```python
from build123d import *

# Parameters (mm, degrees)
SKETCH15_R           = 11.5
BOSS_EXTRUDE8_DEPTH  = 8
BOSS_EXTRUDE9_START  = -8
SKETCH16_R           = 11.5
SKETCH16_R_2         = 11.3
BOSS_EXTRUDE9_DEPTH  = 8
SKETCH17_W           = 10
SKETCH17_H           = 3
BOSS_EXTRUDE10_DEPTH = 8
SKETCH18_W           = 8
SKETCH18_H           = 10
BOSS_EXTRUDE11_DEPTH = 2
SKETCH19_W           = 6
SKETCH19_H           = 3
CUT_EXTRUDE4_DEPTH   = 8
SKETCH20_R           = 2
CUT_EXTRUDE5_DEPTH   = 9
SKETCH21_W           = 29
SKETCH21_H           = 3
BOSS_EXTRUDE12_DEPTH = 7
SKETCH22_R           = 2
CUT_EXTRUDE6_DEPTH   = 7
FILLET1_R            = 5
SKETCH24_R           = 2
CUT_EXTRUDE10_DEPTH  = 8


with BuildPart() as part:
    # Sketch15 → Boss-Extrude8 (new body)
    with BuildSketch(Plane(origin=(3.715547427, 0, 0), x_dir=(0, 0, -1), z_dir=(1, 0, 0))):
        with BuildLine():
            Line((33.146692928, -20.712987114), (4.146692928, -20.712987114))
            Line((4.146692928, -20.712987114), (4.146692928, 9.287012886))
            ThreePointArc((4.146692928, 9.287012886), (18.646692928, 23.787012886), (33.146692928, 9.287012886))
            Line((33.146692928, 9.287012886), (33.146692928, -20.712987114))
        make_face()
        with Locations((18.646692928, 9.287012886)):
            Circle(SKETCH15_R, mode=Mode.SUBTRACT)
    extrude(amount=-BOSS_EXTRUDE8_DEPTH)

    # Sketch16 → Boss-Extrude9 (add)
    with BuildSketch(Plane.ZY.offset(4.284452573).offset(BOSS_EXTRUDE9_START)):
        with Locations((-18.646692928, 9.287012886)):
            Circle(SKETCH16_R)
        with Locations((-18.646692928, 9.287012886)):
            Circle(SKETCH16_R_2, mode=Mode.SUBTRACT)
    extrude(amount=BOSS_EXTRUDE9_DEPTH)

    # Sketch17 → Boss-Extrude10 (add)
    with BuildSketch(Plane.ZY.offset(4.284452573)):
        with Locations((-18.646692928, 23.787012886)):
            Rectangle(SKETCH17_W, SKETCH17_H)
    extrude(amount=-BOSS_EXTRUDE10_DEPTH)

    # Sketch18 → Boss-Extrude11 (add)
    with BuildSketch(Plane(origin=(0, 25.287012886, 0), x_dir=(1, 0, 0), z_dir=(0, 1, 0))):
        with Locations((-0.284452573, 18.646692928)):
            Rectangle(SKETCH18_W, SKETCH18_H)
    extrude(amount=BOSS_EXTRUDE11_DEPTH)

    # Sketch19 → Cut-Extrude4 (cut)
    with BuildSketch(Plane.ZY.offset(4.284452573)):
        with Locations((-18.646692928, 23.787012886)):
            Rectangle(SKETCH19_W, SKETCH19_H)
    extrude(amount=-CUT_EXTRUDE4_DEPTH, mode=Mode.SUBTRACT)

    # Sketch20 → Cut-Extrude5 (cut)
    with BuildSketch(Plane(origin=(0, 27.287012886, 0), x_dir=(1, 0, 0), z_dir=(0, 1, 0))):
        with Locations(Location((-0.284452573, 18.646692928, 0), (0, 0, 270))):
            Circle(SKETCH20_R)
    extrude(amount=-CUT_EXTRUDE5_DEPTH, mode=Mode.SUBTRACT)

    # Sketch21 → Boss-Extrude12 (add)
    with BuildSketch(Plane.ZY.offset(4.284452573)):
        with Locations((-18.646692928, -19.212987114)):
            Rectangle(SKETCH21_W, SKETCH21_H)
    extrude(amount=BOSS_EXTRUDE12_DEPTH)

    # Sketch22 → Cut-Extrude6 (cut)
    with BuildSketch(Plane(origin=(0, -17.712987114, 0), x_dir=(1, 0, 0), z_dir=(0, 1, 0))):
        with Locations(Location((-7.784452573, 11.396692928, 0), (0, 0, 180))):
            Circle(SKETCH22_R)
        with Locations(Location((-7.784452573, 18.646692928, 0), (0, 0, 180))):
            Circle(SKETCH22_R)
        with Locations(Location((-7.784452573, 25.896692928, 0), (0, 0, 180))):
            Circle(SKETCH22_R)
    extrude(amount=-CUT_EXTRUDE6_DEPTH, mode=Mode.SUBTRACT)

    # Fillet1
    fillet1_edges = [part.edges().sort_by_distance(p)[0] for p in [
        (-11.284452573, -19.212987114, -33.146692928),
        (-11.284452573, -19.212987114, -4.146692928),
    ]]
    fillet(fillet1_edges, radius=FILLET1_R)

    # Sketch24 → Cut-Extrude10 (cut)
    with BuildSketch(Plane.ZY.offset(4.284452573)):
        with Locations((-18.646692928, -8.812987114)):
            Circle(SKETCH24_R)
        with Locations((-13.646692928, -8.812987114)):
            Circle(SKETCH24_R)
        with Locations((-23.646692928, -8.812987114)):
            Circle(SKETCH24_R)
        with Locations((-28.646692928, -8.812987114)):
            Circle(SKETCH24_R)
        with Locations((-8.646692928, -8.812987114)):
            Circle(SKETCH24_R)
    extrude(amount=-CUT_EXTRUDE10_DEPTH, mode=Mode.SUBTRACT)


solid = part.part
```
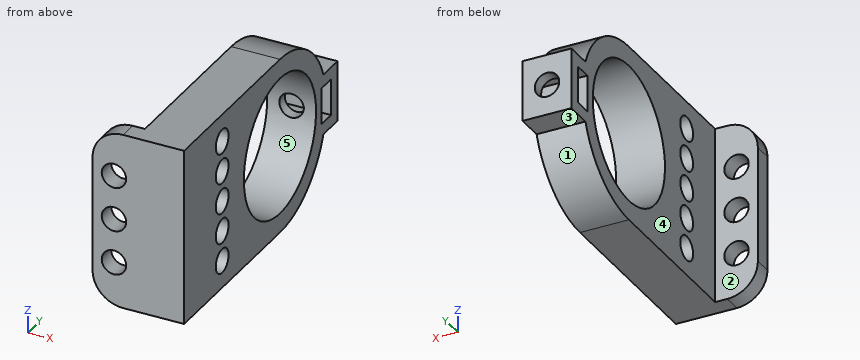
Verification items for the finished model (mm, model axes). Face numbers are marked on the shaded views. A direction names the side the tool comes from. Coordinates: 2 decimals unless noted, no trailing zeros. Write each loop counter-clockwise with the first axis right and the second up, starting at its lowest first coordinate (ties: lowest second). Pieces come first, ordered by that corner, then holes. Notation, with made-up numbers: M 74,41 L 133,41 A11 cw 133,46 Z; hole C -22.5,40 d6. An arc over 180 degrees is marked long. One line per item, written item: value.
Item 1: Section check C-C, the plane x = -1. Record the boundary of the cut face in (y, z), plus the area to 3 significant figures.
Check sheet entries:
outline: M -20.71,-33.15 L 9.29,-33.15 A14.5 ccw 22.9,-23.65 L 27.29,-23.65 L 27.29,-20.51 L 25.29,-20.51 L 25.29,-21.65 L 22.29,-21.65 L 22.29,-20.51 L 20.43,-20.51 A11.3 cw long 20.43,-16.78 L 22.29,-16.78 L 22.29,-15.65 L 25.29,-15.65 L 25.29,-16.78 L 27.29,-16.78 L 27.29,-13.65 L 22.9,-13.65 A14.5 ccw 9.29,-4.15 L -20.71,-4.15 Z; hole C -8.81,-28.65 d4; hole C -8.81,-23.65 d4; hole C -8.81,-18.65 d4; hole C -8.81,-13.65 d4; hole C -8.81,-8.65 d4
area: 742 mm^2
Item 2: Gauge pin test, flat ends, axial feed: pin 1 Ø6.5 at (y, z) = (-8.81, -23.65) entering from -X; pin 2 Ø3.5 at (x, z) = (-7.78, -25.9) entering from +Y; pin 3 Ø5 at (x, z) = (-9, -23.5) entering from +Y; pin 4 Ø3.5 at (x, y) = (1, 25.5) entering from -Z. Record the tip position at first contact, or that the pin passes through.
Check sheet entries:
pin 1: stops at x = -4.28
pin 2: passes through
pin 3: stops at y = -17.71
pin 4: stops at z = -23.65
Item 3: Mould release check, pull along Z, two halves, no side actions. Record for the marked faces 3, 4 and 5: pulls with the +Z half, pulls with the -Z half, needs draft (parallel to the pull), parting line crosses it, or undercut.
Check sheet entries:
face 3: pulls with the -Z half
face 4: needs draft
face 5: undercut
Item 4: Section check D-D, the plane x = -7.25. Record the boundary of the cut face in (y, z).
Check sheet entries:
outline: M -20.71,-33.05 L -17.71,-33.05 L -17.71,-27.82 L -20.71,-27.82 Z; M -20.71,-23.97 L -17.71,-23.97 L -17.71,-20.57 L -20.71,-20.57 Z; M -20.71,-16.72 L -17.71,-16.72 L -17.71,-13.32 L -20.71,-13.32 Z; M -20.71,-9.47 L -17.71,-9.47 L -17.71,-4.24 L -20.71,-4.24 Z
Item 5: Section check A-A, the plane y = 24. Record the boundary of the cut face in (x, z), plus the area to 3 significant figures.
Check sheet entries:
outline: M -4.28,-23.65 L 3.72,-23.65 L 3.72,-21.65 L -4.28,-21.65 Z; M -4.28,-15.65 L 3.72,-15.65 L 3.72,-13.65 L -4.28,-13.65 Z
area: 32.0 mm^2
Item 6: Scan lines: line 1 along Z through (x, y) = (2.75, 23); line 2 along Y through (x, z) = (-2.25, -19.5); line 3 along Z through (x, y) = (3, 6.5). Record each from-to range of solid material in increasing order.
Check sheet entries:
line 1: z = -23.65 to -21.65, -15.65 to -13.65
line 2: y = -20.71 to -10.62, -7 to -1.98, 20.55 to 22.29, 25.29 to 27.29
line 3: z = -33.15 to -29.6, -7.7 to -4.15
Item 7: Access from +Z, -Z, +X, -X, +Y, -Y to the whole of each face (thin tool, end or side, straight path). Record for the marked faces 1 and 2.
Check sheet entries:
face 1: -Z, +X, -X, +Y
face 2: +Z, -Z, -X, +Y
Item 8: Section check B-B, the plane z = -15. Record the boundary of the cut face in (x, y).
Check sheet entries:
outline: M -11.28,-20.71 L 3.72,-20.71 L 3.72,-10.29 L -4.28,-10.29 L -4.28,-17.71 L -11.28,-17.71 Z; M -4.28,-7.34 L 3.72,-7.34 L 3.72,-1.41 L -4.28,-1.41 Z; M -4.28,19.98 L 3.72,19.98 L 3.72,27.29 L -4.28,27.29 Z
